Could you check a few things on this model? Use its own coordinates, in mm. Face numbers are marked on the shaded views. A direction names the side the tool comes from. Round coordinates to 2 decimals unless told otherwise and drop trailing zeros. Loops run counter-clockwise (first coordinate to the right, second up) from the corner with the lowest first, then second, coordinate; pieces in that order, holes last. Notation, with made-up numbers: (61.5, 40.5) -> (78.5, 40.5) arc R19 ccw to (78.5, 47.5) -> close; hole circle Ø4 at (71.5, -11.5). An arc over 180 degrees is marked (long way). Put each result on its own line as item: value. Start each with the question number.
1. Imagine slicing it at A-A, the plane y = 5. Please give me the cut outline in (x, z).
2. Imagine slicing it at B-B, the plane x = -31. Please give me the cut outline in (y, z), and give its area (3 significant figures).
3. I'm going to push flat-ended pins straight in: P1, Ø1, axis at x = -5.5, z = 24, coming from the -Y side; P2, Ø1.5, axis at x = -33.5, z = 7.5, coming from the -Y side. Where does each tip first touch, or does it pass through?
4. Which directions (+Z, -Z, +X, -X, +Y, -Y) give clear straight access to the entire face, cutting with the end or side of a thin tool? Please do the marked faces 4 and 5.
5. Imagine slicing it at D-D, the plane y = 9.5. Please give me the cut outline in (x, z).
6. Imagine slicing it at C-C, the plane z = 32.5. Please give me the cut outline in (x, y), and give its area (3 significant figures).
7. If we mould it in two halves opening along Z, with no side actions, what happens to the marked faces 1, 2 and 3? For each: pulls with the +Z half, pulls with the -Z half, needs draft (parallel to the pull), parting line crosses it, or undercut.
8. I need wall thicknesses on line 1 (X direction, y = 0, z = 14.5); line 2 (Y direction, x = 1, z = -3). Which ranges of each line are inside material? Lowest first, please. Write a range as [from, to].
```python
from build123d import *

# Parameters (mm, degrees)
BOSS_EXTRUDE1_DEPTH = 42.5
SHELL1_T            = -2


with BuildPart() as part:
    # Sketch3 → Boss-Extrude1 (new, symmetric)
    with BuildSketch(Plane.XY):
        with BuildLine():
            Line((-32.5, 16.5), (32.5, 16.5))
            ThreePointArc((32.5, 16.5), (39.571067812, 13.571067812), (42.5, 6.5))
            Line((42.5, 6.5), (42.5, -16.5))
            Line((42.5, -16.5), (-42.5, -16.5))
            Line((-42.5, -16.5), (-42.5, 6.5))
            ThreePointArc((-42.5, 6.5), (-39.571067812, 13.571067812), (-32.5, 16.5))
        make_face()
    extrude(amount=BOSS_EXTRUDE1_DEPTH, both=True)

    # Shell1
    shell1_openings = [part.faces().sort_by_distance(p)[0] for p in [
        (0, -16.5, 0),
    ]]
    offset(amount=SHELL1_T, openings=shell1_openings, kind=Kind.INTERSECTION)


solid = part.part
```
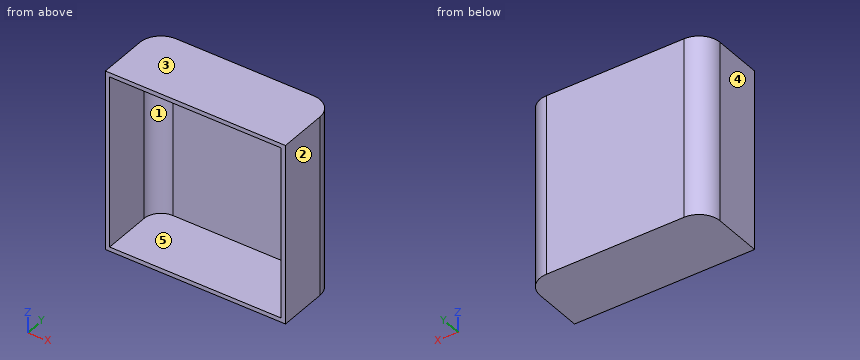
Entries:
1. outline: (-42.5, -42.5) -> (42.5, -42.5) -> (42.5, 42.5) -> (-42.5, 42.5) -> close; hole (-40.5, -40.5) -> (40.5, -40.5) -> (40.5, 40.5) -> (-40.5, 40.5) -> close
2. outline: (-16.5, -42.5) -> (16.5, -42.5) -> (16.5, 42.5) -> (-16.5, 42.5) -> (-16.5, 40.5) -> (14.5, 40.5) -> (14.5, -40.5) -> (-16.5, -40.5) -> close
2. area: 294 mm^2
3. P1: y = 14.5
3. P2: y = 14.31
4. face 4: +Z, -Z, -X, +Y, -Y
4. face 5: -Y
5. outline: (-42.04, -42.5) -> (42.04, -42.5) -> (42.04, 42.5) -> (-42.04, 42.5) -> close; hole (-39.92, -40.5) -> (39.92, -40.5) -> (39.92, 40.5) -> (-39.92, 40.5) -> close
6. outline: (-42.5, -16.5) -> (-40.5, -16.5) -> (-40.5, 6.5) arc R8 cw to (-32.5, 14.5) -> (32.5, 14.5) arc R8 cw to (40.5, 6.5) -> (40.5, -16.5) -> (42.5, -16.5) -> (42.5, 6.5) arc R10 ccw to (32.5, 16.5) -> (-32.5, 16.5) arc R10 ccw to (-42.5, 6.5) -> close
6. area: 279 mm^2
7. face 1: undercut
7. face 2: needs draft
7. face 3: pulls with the +Z half
8. line 1: [-42.5, -40.5], [40.5, 42.5]
8. line 2: [14.5, 16.5]
